from build123d import *

# Parameters (mm, degrees)
SKETCH1_W                       = 140
SKETCH1_H                       = 80
BOSS_EXTRUDE1_DEPTH             = 2
SKETCH3_W                       = 126
SKETCH3_H                       = 66
SKETCH2_W                       = 140
SKETCH2_H                       = 80
CHAMFER2_SIZE                   = 2
SKETCH4_W                       = 8
SKETCH4_H                       = 10
BOSS_EXTRUDE2_DEPTH             = 7
SKETCH5_R                       = 2.05
CUT_EXTRUDE1_DEPTH              = 133.9000001
SKETCH6_W                       = 107.8
SKETCH6_H                       = 64
CUT_EXTRUDE2_DEPTH              = 5
SKIZZE1_R                       = 2.15
SCHNITT_LINEAR_AUSTRAGEN2_DEPTH = 10


with BuildPart() as part:
    # Sketch1 → Boss-Extrude1 (new body)
    with BuildSketch(Plane(origin=(0, 0, 0), x_dir=(1, 0, 0), z_dir=(0, 1, 0))):
        Rectangle(SKETCH1_W, SKETCH1_H)
    extrude(amount=BOSS_EXTRUDE1_DEPTH)

    # Sketch3 → Loft1 section 0
    with BuildSketch(Plane(origin=(0, 7, 0), x_dir=(1, 0, 0), z_dir=(0, 1, 0))):
        Rectangle(SKETCH3_W, SKETCH3_H)
    # Sketch2 → Loft1 section 1
    with BuildSketch(Plane(origin=(0, 2, 0), x_dir=(1, 0, 0), z_dir=(0, 1, 0))):
        Rectangle(SKETCH2_W, SKETCH2_H)
    loft()

    # Chamfer2
    chamfer2_edges = [part.edges().sort_by_distance(p)[0] for p in [
        (70, 1, 40),
        (-70, 1, 40),
        (-70, 1, -40),
        (70, 1, -40),
    ]]
    chamfer(chamfer2_edges, length=CHAMFER2_SIZE)

    # Sketch4 → Boss-Extrude2 (add)
    with BuildSketch(Plane.XZ):
        with Locations((-58.9, 20)):
            Rectangle(SKETCH4_W, SKETCH4_H)
        with Locations((-58.9, -20)):
            Rectangle(SKETCH4_W, SKETCH4_H)
        with Locations((58.9, -20)):
            Rectangle(SKETCH4_W, SKETCH4_H)
        with Locations((58.9, 20)):
            Rectangle(SKETCH4_W, SKETCH4_H)
    extrude(amount=BOSS_EXTRUDE2_DEPTH)

    # Sketch5 → Cut-Extrude1 (cut, through all)
    with BuildSketch(Plane.ZY.offset(62.9)):
        with Locations((-20, -3.5)):
            Circle(SKETCH5_R)
        with Locations((20, -3.5)):
            Circle(SKETCH5_R)
    extrude(amount=-CUT_EXTRUDE1_DEPTH, mode=Mode.SUBTRACT)

    # Sketch6 → Cut-Extrude2 (cut)
    with BuildSketch(Plane.XZ):
        Rectangle(SKETCH6_W, SKETCH6_H)
    extrude(amount=-CUT_EXTRUDE2_DEPTH, mode=Mode.SUBTRACT)

    # Skizze1 → Schnitt-Linear austragen2 (cut)
    with BuildSketch(Plane(origin=(0, 7, 0), x_dir=(1, 0, 0), z_dir=(0, 1, 0))):
        with Locations((-50, -25)):
            Circle(SKIZZE1_R)
        with Locations((-40, -25)):
            Circle(SKIZZE1_R)
        with Locations((-30, -25)):
            Circle(SKIZZE1_R)
        with Locations((-20, -25)):
            Circle(SKIZZE1_R)
        with Locations((-10, -25)):
            Circle(SKIZZE1_R)
        with Locations((0, -25)):
            Circle(SKIZZE1_R)
        with Locations((10, -25)):
            Circle(SKIZZE1_R)
        with Locations((20, -25)):
            Circle(SKIZZE1_R)
        with Locations((30, -25)):
            Circle(SKIZZE1_R)
        with Locations((40, -25)):
            Circle(SKIZZE1_R)
        with Locations((50, -25)):
            Circle(SKIZZE1_R)
        with Locations((-40, -15)):
            Circle(SKIZZE1_R)
        with Locations((-30, -15)):
            Circle(SKIZZE1_R)
        with Locations((-20, -15)):
            Circle(SKIZZE1_R)
        with Locations((-10, -15)):
            Circle(SKIZZE1_R)
        with Locations((0, -15)):
            Circle(SKIZZE1_R)
        with Locations((10, -15)):
            Circle(SKIZZE1_R)
        with Locations((20, -15)):
            Circle(SKIZZE1_R)
        with Locations((30, -15)):
            Circle(SKIZZE1_R)
        with Locations((40, -15)):
            Circle(SKIZZE1_R)
        with Locations((50, -15)):
            Circle(SKIZZE1_R)
        with Locations((-40, -5)):
            Circle(SKIZZE1_R)
        with Locations((-30, -5)):
            Circle(SKIZZE1_R)
        with Locations((-20, -5)):
            Circle(SKIZZE1_R)
        with Locations((-10, -5)):
            Circle(SKIZZE1_R)
        with Locations((0, -5)):
            Circle(SKIZZE1_R)
        with Locations((10, -5)):
            Circle(SKIZZE1_R)
        with Locations((20, -5)):
            Circle(SKIZZE1_R)
        with Locations((30, -5)):
            Circle(SKIZZE1_R)
        with Locations((40, -5)):
            Circle(SKIZZE1_R)
        with Locations((50, -5)):
            Circle(SKIZZE1_R)
        with Locations((-40, 5)):
            Circle(SKIZZE1_R)
        with Locations((-30, 5)):
            Circle(SKIZZE1_R)
        with Locations((-20, 5)):
            Circle(SKIZZE1_R)
        with Locations((-10, 5)):
            Circle(SKIZZE1_R)
        with Locations((0, 5)):
            Circle(SKIZZE1_R)
        with Locations((10, 5)):
            Circle(SKIZZE1_R)
        with Locations((20, 5)):
            Circle(SKIZZE1_R)
        with Locations((30, 5)):
            Circle(SKIZZE1_R)
        with Locations((40, 5)):
            Circle(SKIZZE1_R)
        with Locations((50, 5)):
            Circle(SKIZZE1_R)
        with Locations((-40, 15)):
            Circle(SKIZZE1_R)
        with Locations((-30, 15)):
            Circle(SKIZZE1_R)
        with Locations((-20, 15)):
            Circle(SKIZZE1_R)
        with Locations((-10, 15)):
            Circle(SKIZZE1_R)
        with Locations((0, 15)):
            Circle(SKIZZE1_R)
        with Locations((10, 15)):
            Circle(SKIZZE1_R)
        with Locations((20, 15)):
            Circle(SKIZZE1_R)
        with Locations((30, 15)):
            Circle(SKIZZE1_R)
        with Locations((40, 15)):
            Circle(SKIZZE1_R)
        with Locations((50, 15)):
            Circle(SKIZZE1_R)
        with Locations((-40, 25)):
            Circle(SKIZZE1_R)
        with Locations((-30, 25)):
            Circle(SKIZZE1_R)
        with Locations((-20, 25)):
            Circle(SKIZZE1_R)
        with Locations((-10, 25)):
            Circle(SKIZZE1_R)
        with Locations((0, 25)):
            Circle(SKIZZE1_R)
        with Locations((10, 25)):
            Circle(SKIZZE1_R)
        with Locations((20, 25)):
            Circle(SKIZZE1_R)
        with Locations((30, 25)):
            Circle(SKIZZE1_R)
        with Locations((40, 25)):
            Circle(SKIZZE1_R)
        with Locations((50, 25)):
            Circle(SKIZZE1_R)
        with Locations((-50, -15)):
            Circle(SKIZZE1_R)
        with Locations((-50, -5)):
            Circle(SKIZZE1_R)
        with Locations((-50, 5)):
            Circle(SKIZZE1_R)
        with Locations((-50, 15)):
            Circle(SKIZZE1_R)
        with Locations((-50, 25)):
            Circle(SKIZZE1_R)
    extrude(amount=-SCHNITT_LINEAR_AUSTRAGEN2_DEPTH, mode=Mode.SUBTRACT)


solid = part.part
For this review, take the finished solid that the model builds, in its own axes (mm). A direction names the side the tool comes from. Coordinates: 2 decimals unless noted, no trailing zeros. Use one line per item in the form item = value.
Q1. For probe 1 along Z at (x, y) = (34.5, 0.75); probe 2 along X at (y, z) = (-4, 16); probe 3 along Y at (x, z) = (11.5, 28), list the stretches that pass through material, from the lowest coordinate up. Write a range as from..to.
Checked values:
probe_1 = -40..-32, 32..40
probe_2 = -62.9..-54.9, 54.9..62.9
probe_3 = 5..7
Q2. For faces 5 (the flat face through (-1, 2, -32)), 6 (the cylindrical face through (-49.01, 6.01, -13.09)), 7 (the flat face through (62.9, -3.5, -22.3)), 8 (the flat face through (54.9, -3.5, -22.3)), list the 3-axis set-ups (+Z, -Z, +X, -X, +Y, -Y) from which the entire face can be reached by the end or side of a thin tool; tool diameter is ignored.
Checked values:
face_5 = -Y
face_6 = +Y, -Y
face_7 = +Z, -Z, +X, -Y
face_8 = +Z, -Z, -Y
Q3. Consider section A-A (y = -3.5). Give the number of separate pieces and of enclosed holes in the cut face, then the cut area to 3 significant figures.
Checked values:
separate_pieces = 8
enclosed_holes = 0
area = 189 mm2
Q4. For P1, Ø4.5, axis at y = -3.5, z = 20, coming from the -X side; P2, Ø3.5, axis at x = -50, z = 5, coming from the -Y side; P3, Ø6, axis at x = 8, z = -4, coming from the -Y side; P4, Ø10, axis at x = -32.5, z = -29, coming from the -Y side, all flat-tipped, find the tip position at first contact; note any pin that passes through.
Checked values:
P1 = -62.9
P2 = through
P3 = 5
P4 = 0
Q5. Draft analysis for pull direction Z (two halves, no side actions). For faces 1 (the flat face through (-59, -3, -25)), 2 (the cylindrical face through (30.99, 6.01, 26.91)), 3 (the flat face through (-59, -7, -20)), 4 (the cylindrical face through (19.72, 6.01, -7.13)), state which applies: +Z half, -Z half, draft (parallel to the pull), parting line (faces both ways), or undercut.
Checked values:
face_1 = -Z half
face_2 = undercut
face_3 = draft
face_4 = undercut
